```python
from build123d import *

# Parameters (mm, degrees)
SKETCH1_W           = 30.65
SKETCH1_H           = 12.1
BOSS_EXTRUDE1_DEPTH = 12.4
SKETCH2_R           = 2
SKETCH2_W           = 1.2
SKETCH2_H           = 4.3
CUT_EXTRUDE1_DEPTH  = 10
SKETCH3_R           = 0.425
CUT_EXTRUDE2_DEPTH  = 12.4
SKETCH4_W           = 30.65
SKETCH4_H           = 1.9
SKETCH4_W_2         = 17.6
SKETCH4_H_2         = 0.8
SKETCH4_W_3         = 6.5
SKETCH4_H_3         = 5.95
CUT_EXTRUDE3_DEPTH  = 10.1
CUT_EXTRUDE4_REACH  = 21.537
SKETCH6_W           = 6.5
SKETCH6_H           = 8.2
SKETCH7_W           = 15.65
SKETCH7_H           = 6.6
CUT_EXTRUDE5_DEPTH  = 6.35
CUT_EXTRUDE6_REACH  = 21.019
FILLET1_R           = 1.5
SKETCH10_W          = 3.4
SKETCH10_H          = 3
CUT_EXTRUDE7_DEPTH  = 4.8
SKETCH11_W          = 3.4
SKETCH11_H          = 3
CUT_EXTRUDE8_DEPTH  = 9.5
FILLET2_R           = 1.5
SKETCH12_R          = 2.5
CUT_EXTRUDE9_DEPTH  = 0.5
CUT_EXTRUDE10_REACH = 22.15
SKETCH13_W          = 0.8
SKETCH13_H          = 1.6
SKETCH13_H_2        = 4.5
FILLET3_R           = 0.25
SKETCH14_R          = 0.725
CUT_EXTRUDE11_DEPTH = 1


with BuildPart() as part:
    # Sketch1 → Boss-Extrude1 (new body)
    with BuildSketch(Plane(origin=(0, 0, 0), x_dir=(1, 0, 0), z_dir=(0, 1, 0))):
        Rectangle(SKETCH1_W, SKETCH1_H)
    extrude(amount=BOSS_EXTRUDE1_DEPTH)

    # Sketch2 → Cut-Extrude1 (cut)
    with BuildSketch(Plane.XY.offset(6.05)):
        with Locations((-12.5, 6.4)):
            Circle(SKETCH2_R)
        with Locations(Location((12.5, 6.4, 0), (0, 0, 180))):
            Circle(SKETCH2_R)
        with Locations((-7.3, 6.2)):
            Rectangle(SKETCH2_W, SKETCH2_H)
        with Locations((7.3, 6.2)):
            Rectangle(SKETCH2_W, SKETCH2_H)
    extrude(amount=-CUT_EXTRUDE1_DEPTH, mode=Mode.SUBTRACT)

    # Sketch3 → Cut-Extrude2 (cut)
    with BuildSketch(Plane.XY.offset(6.05)):
        with Locations((-5.1, 7.675)):
            Circle(SKETCH3_R)
        with Locations((-2.55, 7.675)):
            Circle(SKETCH3_R)
        with Locations((0, 7.675)):
            Circle(SKETCH3_R)
        with Locations((2.55, 7.675)):
            Circle(SKETCH3_R)
        with Locations((5.1, 7.675)):
            Circle(SKETCH3_R)
        with Locations((-3.825, 4.725)):
            Circle(SKETCH3_R)
        with Locations((-1.275, 4.725)):
            Circle(SKETCH3_R)
        with Locations((1.275, 4.725)):
            Circle(SKETCH3_R)
        with Locations((3.825, 4.725)):
            Circle(SKETCH3_R)
    extrude(amount=-CUT_EXTRUDE2_DEPTH, mode=Mode.SUBTRACT)

    # Sketch4 → Cut-Extrude3 (cut)
    with BuildSketch(Plane(origin=(0, 0, -6.05), x_dir=(-1, 0, 0), z_dir=(0, 0, -1))):
        with Locations((0, 11.45)):
            Rectangle(SKETCH4_W, SKETCH4_H)
        with Locations((0, 0.4)):
            Rectangle(SKETCH4_W_2, SKETCH4_H_2)
        with Locations((12.075, 5.875)):
            Rectangle(SKETCH4_W_3, SKETCH4_H_3)
        with Locations((-12.075, 5.875)):
            Rectangle(SKETCH4_W_3, SKETCH4_H_3)
    extrude(amount=-CUT_EXTRUDE3_DEPTH, mode=Mode.SUBTRACT)

    # Sketch6 → Cut-Extrude4 (cut, up to next)
    with BuildSketch(Plane(origin=(0, 10.5, 0), x_dir=(1, 0, 0), z_dir=(0, 1, 0)), mode=Mode.PRIVATE) as cut_extrude4_sk1:
        with Locations((12.075, 1.95)):
            Rectangle(SKETCH6_W, SKETCH6_H)
    cut_extrude4_tool1 = extrude(cut_extrude4_sk1.sketch, amount=-CUT_EXTRUDE4_REACH, mode=Mode.PRIVATE) & part.part
    # Sketch6 → Cut-Extrude4 (cut, up to next)
    with BuildSketch(Plane(origin=(0, 10.5, 0), x_dir=(1, 0, 0), z_dir=(0, 1, 0)), mode=Mode.PRIVATE) as cut_extrude4_sk2:
        with Locations((-12.075, 1.95)):
            Rectangle(SKETCH6_W, SKETCH6_H)
    cut_extrude4_tool2 = extrude(cut_extrude4_sk2.sketch, amount=-CUT_EXTRUDE4_REACH, mode=Mode.PRIVATE) & part.part
    add(cut_extrude4_tool1.solids().sort_by_distance((12.075, 10.5, -1.95))[0], mode=Mode.SUBTRACT)
    add(cut_extrude4_tool2.solids().sort_by_distance((-12.075, 10.5, -1.95))[0], mode=Mode.SUBTRACT)

    # Sketch7 → Cut-Extrude5 (cut)
    with BuildSketch(Plane(origin=(0, 0, -6.05), x_dir=(-1, 0, 0), z_dir=(0, 0, -1))):
        with Locations((0, 6.2)):
            Rectangle(SKETCH7_W, SKETCH7_H)
    extrude(amount=-CUT_EXTRUDE5_DEPTH, mode=Mode.SUBTRACT)

    # Sketch8 → Cut-Extrude6 (cut, up to next)
    with BuildSketch(Plane(origin=(0, 2.9, 0), x_dir=(1, 0, 0), z_dir=(0, 1, 0)), mode=Mode.PRIVATE) as cut_extrude6_sk1:
        with BuildLine():
            Line((-10.795, 3.45), (-10.795, 1.25))
            ThreePointArc((-10.795, 1.25), (-12.495, -0.45), (-14.195, 1.25))
            Line((-14.195, 1.25), (-14.195, 3.45))
            ThreePointArc((-14.195, 3.45), (-12.495, 5.15), (-10.795, 3.45))
        make_face()
    cut_extrude6_tool1 = extrude(cut_extrude6_sk1.sketch, amount=-CUT_EXTRUDE6_REACH, mode=Mode.PRIVATE) & part.part
    # Sketch8 → Cut-Extrude6 (cut, up to next)
    with BuildSketch(Plane(origin=(0, 2.9, 0), x_dir=(1, 0, 0), z_dir=(0, 1, 0)), mode=Mode.PRIVATE) as cut_extrude6_sk2:
        with BuildLine():
            Line((10.795, 3.45), (10.795, 1.25))
            ThreePointArc((10.795, 1.25), (12.495, -0.45), (14.195, 1.25))
            Line((14.195, 1.25), (14.195, 3.45))
            ThreePointArc((14.195, 3.45), (12.495, 5.15), (10.795, 3.45))
        make_face()
    cut_extrude6_tool2 = extrude(cut_extrude6_sk2.sketch, amount=-CUT_EXTRUDE6_REACH, mode=Mode.PRIVATE) & part.part
    add(cut_extrude6_tool1.solids().sort_by_distance((-12.495, 2.9, -2.35))[0], mode=Mode.SUBTRACT)
    add(cut_extrude6_tool2.solids().sort_by_distance((12.495, 2.9, -2.35))[0], mode=Mode.SUBTRACT)

    # Fillet1
    fillet1_edges = [part.edges().sort_by_distance(p)[0] for p in [
        (8.825, 10.5, -1.95),
        (-8.825, 10.5, -1.95),
    ]]
    fillet(fillet1_edges, radius=FILLET1_R)

    # Sketch10 → Cut-Extrude7 (cut)
    with BuildSketch(Plane(origin=(0, 0, -6.05), x_dir=(-1, 0, 0), z_dir=(0, 0, -1))):
        with Locations((-12.5, 2.9)):
            Rectangle(SKETCH10_W, SKETCH10_H)
    cut_extrude7 = extrude(amount=-CUT_EXTRUDE7_DEPTH, mode=Mode.SUBTRACT)

    # Sketch11 → Cut-Extrude8 (cut)
    with BuildSketch(Plane.XY.offset(6.05)):
        with Locations((12.5, 0)):
            Rectangle(SKETCH11_W, SKETCH11_H)
    cut_extrude8 = extrude(amount=-CUT_EXTRUDE8_DEPTH, mode=Mode.SUBTRACT)

    # Mirror3: Cut-Extrude7, Cut-Extrude8 across plane
    add(cut_extrude7.mirror(Plane(origin=(0, 0, 0), x_dir=(0, 0, 1), z_dir=(1, 0, 0))), mode=Mode.SUBTRACT)
    add(cut_extrude8.mirror(Plane(origin=(0, 0, 0), x_dir=(0, 0, 1), z_dir=(1, 0, 0))), mode=Mode.SUBTRACT)

    # Fillet2
    fillet2_edges = [part.edges().sort_by_distance(p)[0] for p in [
        (15.325, 12.4, 5.05),
        (-15.325, 12.4, 5.05),
    ]]
    fillet(fillet2_edges, radius=FILLET2_R)

    # Sketch12 → Cut-Extrude9 (cut)
    with BuildSketch(Plane.XY.offset(6.05)):
        with Locations((-12.5, 6.4)):
            Circle(SKETCH12_R)
        with Locations((12.5, 6.4)):
            Circle(SKETCH12_R)
    extrude(amount=-CUT_EXTRUDE9_DEPTH, mode=Mode.SUBTRACT)

    # Sketch13 → Cut-Extrude10 (cut, up to next)
    with BuildSketch(Plane.XZ.offset(-0.8), mode=Mode.PRIVATE) as cut_extrude10_sk1:
        with Locations((5.095, -5.25)):
            Rectangle(SKETCH13_W, SKETCH13_H)
    cut_extrude10_tool1 = extrude(cut_extrude10_sk1.sketch, amount=-CUT_EXTRUDE10_REACH, mode=Mode.PRIVATE) & part.part
    # Sketch13 → Cut-Extrude10 (cut, up to next)
    with BuildSketch(Plane.XZ.offset(-0.8), mode=Mode.PRIVATE) as cut_extrude10_sk2:
        with Locations((1.275, -3.8)):
            Rectangle(SKETCH13_W, SKETCH13_H_2)
    cut_extrude10_tool2 = extrude(cut_extrude10_sk2.sketch, amount=-CUT_EXTRUDE10_REACH, mode=Mode.PRIVATE) & part.part
    # Sketch13 → Cut-Extrude10 (cut, up to next)
    with BuildSketch(Plane.XZ.offset(-0.8), mode=Mode.PRIVATE) as cut_extrude10_sk3:
        with Locations((3.825, -3.8)):
            Rectangle(SKETCH13_W, SKETCH13_H_2)
    cut_extrude10_tool3 = extrude(cut_extrude10_sk3.sketch, amount=-CUT_EXTRUDE10_REACH, mode=Mode.PRIVATE) & part.part
    # Sketch13 → Cut-Extrude10 (cut, up to next)
    with BuildSketch(Plane.XZ.offset(-0.8), mode=Mode.PRIVATE) as cut_extrude10_sk4:
        with Locations((2.545, -5.25)):
            Rectangle(SKETCH13_W, SKETCH13_H)
    cut_extrude10_tool4 = extrude(cut_extrude10_sk4.sketch, amount=-CUT_EXTRUDE10_REACH, mode=Mode.PRIVATE) & part.part
    # Sketch13 → Cut-Extrude10 (cut, up to next)
    with BuildSketch(Plane.XZ.offset(-0.8), mode=Mode.PRIVATE) as cut_extrude10_sk5:
        with Locations((-1.275, -3.8)):
            Rectangle(SKETCH13_W, SKETCH13_H_2)
    cut_extrude10_tool5 = extrude(cut_extrude10_sk5.sketch, amount=-CUT_EXTRUDE10_REACH, mode=Mode.PRIVATE) & part.part
    # Sketch13 → Cut-Extrude10 (cut, up to next)
    with BuildSketch(Plane.XZ.offset(-0.8), mode=Mode.PRIVATE) as cut_extrude10_sk6:
        with Locations((-0.005, -5.25)):
            Rectangle(SKETCH13_W, SKETCH13_H)
    cut_extrude10_tool6 = extrude(cut_extrude10_sk6.sketch, amount=-CUT_EXTRUDE10_REACH, mode=Mode.PRIVATE) & part.part
    # Sketch13 → Cut-Extrude10 (cut, up to next)
    with BuildSketch(Plane.XZ.offset(-0.8), mode=Mode.PRIVATE) as cut_extrude10_sk7:
        with Locations((-3.825, -3.8)):
            Rectangle(SKETCH13_W, SKETCH13_H_2)
    cut_extrude10_tool7 = extrude(cut_extrude10_sk7.sketch, amount=-CUT_EXTRUDE10_REACH, mode=Mode.PRIVATE) & part.part
    # Sketch13 → Cut-Extrude10 (cut, up to next)
    with BuildSketch(Plane.XZ.offset(-0.8), mode=Mode.PRIVATE) as cut_extrude10_sk8:
        with Locations((-2.555, -5.25)):
            Rectangle(SKETCH13_W, SKETCH13_H)
    cut_extrude10_tool8 = extrude(cut_extrude10_sk8.sketch, amount=-CUT_EXTRUDE10_REACH, mode=Mode.PRIVATE) & part.part
    # Sketch13 → Cut-Extrude10 (cut, up to next)
    with BuildSketch(Plane.XZ.offset(-0.8), mode=Mode.PRIVATE) as cut_extrude10_sk9:
        with Locations((-5.095, -5.25)):
            Rectangle(SKETCH13_W, SKETCH13_H)
    cut_extrude10_tool9 = extrude(cut_extrude10_sk9.sketch, amount=-CUT_EXTRUDE10_REACH, mode=Mode.PRIVATE) & part.part
    add(cut_extrude10_tool1.solids().sort_by_distance((5.095, 0.8, -5.25))[0], mode=Mode.SUBTRACT)
    add(cut_extrude10_tool2.solids().sort_by_distance((1.275, 0.8, -3.8))[0], mode=Mode.SUBTRACT)
    add(cut_extrude10_tool3.solids().sort_by_distance((3.825, 0.8, -3.8))[0], mode=Mode.SUBTRACT)
    add(cut_extrude10_tool4.solids().sort_by_distance((2.545, 0.8, -5.25))[0], mode=Mode.SUBTRACT)
    add(cut_extrude10_tool5.solids().sort_by_distance((-1.275, 0.8, -3.8))[0], mode=Mode.SUBTRACT)
    add(cut_extrude10_tool6.solids().sort_by_distance((-0.005, 0.8, -5.25))[0], mode=Mode.SUBTRACT)
    add(cut_extrude10_tool7.solids().sort_by_distance((-3.825, 0.8, -3.8))[0], mode=Mode.SUBTRACT)
    add(cut_extrude10_tool8.solids().sort_by_distance((-2.555, 0.8, -5.25))[0], mode=Mode.SUBTRACT)
    add(cut_extrude10_tool9.solids().sort_by_distance((-5.095, 0.8, -5.25))[0], mode=Mode.SUBTRACT)

    # Fillet3
    # the kernel refuses this fillet: 0.25 mm, written as the material it takes off along each edge
    with BuildSketch(Plane(origin=(5.495, 0.175, -6.05), x_dir=(1, 0, 0), z_dir=(0, 1, 0))) as fillet3_piece_1:
        with BuildLine():
            CenterArc((FILLET3_R, -FILLET3_R), FILLET3_R, 90, 90)
            Line((0, -FILLET3_R), (0, 0))
            Line((0, 0), (FILLET3_R, 0))
        make_face()
    extrude(amount=3.35, mode=Mode.SUBTRACT)
    with BuildSketch(Plane(origin=(4.695, 0.175, -6.05), x_dir=(-1, 0, 0), z_dir=(0, 1, 0)), Plane(origin=(-4.225, 0.175, -6.05), x_dir=(-1, 0, 0), z_dir=(0, 1, 0)), Plane(origin=(-3.425, 0.175, -6.05), x_dir=(0, 0, 1), z_dir=(0, 1, 0)), Plane(origin=(-2.955, 0.175, -6.05), x_dir=(-1, 0, 0), z_dir=(0, 1, 0)), Plane(origin=(-2.155, 0.175, -6.05), x_dir=(0, 0, 1), z_dir=(0, 1, 0)), Plane(origin=(-1.675, 0.175, -6.05), x_dir=(-1, 0, 0), z_dir=(0, 1, 0)), Plane(origin=(-0.875, 0.175, -6.05), x_dir=(0, 0, 1), z_dir=(0, 1, 0)), Plane(origin=(-0.405, 0.175, -6.05), x_dir=(-1, 0, 0), z_dir=(0, 1, 0)), Plane(origin=(0.395, 0.175, -6.05), x_dir=(0, 0, 1), z_dir=(0, 1, 0)), Plane(origin=(0.875, 0.175, -6.05), x_dir=(-1, 0, 0), z_dir=(0, 1, 0)), Plane(origin=(1.675, 0.175, -6.05), x_dir=(0, 0, 1), z_dir=(0, 1, 0)), Plane(origin=(-5.495, 0.175, -6.05), x_dir=(-1, 0, 0), z_dir=(0, 1, 0)), Plane(origin=(-4.695, 0.175, -6.05), x_dir=(0, 0, 1), z_dir=(0, 1, 0)), Plane(origin=(3.425, 0.175, -6.05), x_dir=(-1, 0, 0), z_dir=(0, 1, 0)), Plane(origin=(4.225, 0.175, -6.05), x_dir=(0, 0, 1), z_dir=(0, 1, 0)), Plane(origin=(2.145, 0.175, -6.05), x_dir=(-1, 0, 0), z_dir=(0, 1, 0)), Plane(origin=(2.945, 0.175, -6.05), x_dir=(0, 0, 1), z_dir=(0, 1, 0))) as fillet3_piece_2:
        with BuildLine():
            CenterArc((FILLET3_R, FILLET3_R), FILLET3_R, 180, 90)
            Line((0, FILLET3_R), (0, 0))
            Line((0, 0), (FILLET3_R, 0))
        make_face()
    extrude(amount=3.35, mode=Mode.SUBTRACT)

    # Sketch14 → Cut-Extrude11 (cut)
    with BuildSketch(Plane(origin=(0, 0, 0.3), x_dir=(-1, 0, 0), z_dir=(0, 0, -1))):
        with Locations((-2.55, 7.675)):
            Circle(SKETCH14_R)
        with Locations((-5.1, 7.675)):
            Circle(SKETCH14_R)
        with Locations((0, 7.675)):
            Circle(SKETCH14_R)
        with Locations((2.55, 7.675)):
            Circle(SKETCH14_R)
        with Locations((5.1, 7.675)):
            Circle(SKETCH14_R)
        with Locations((3.825, 4.725)):
            Circle(SKETCH14_R)
        with Locations((1.275, 4.725)):
            Circle(SKETCH14_R)
        with Locations((-1.275, 4.725)):
            Circle(SKETCH14_R)
        with Locations((-3.825, 4.725)):
            Circle(SKETCH14_R)
    extrude(amount=-CUT_EXTRUDE11_DEPTH, mode=Mode.SUBTRACT)


solid = part.part
```
Input: part model. Units: mm. Frame: model coordinates. A direction names the side the tool comes from. Round coordinates to 2 decimals unless told otherwise and drop trailing zeros. Loops run counter-clockwise (first coordinate to the right, second up) from the corner with the lowest first, then second, coordinate; pieces in that order, holes last. Notation, with made-up numbers: (18, 48.5) -> (24, 48.5) arc R18 ccw to (24, 66.5) -> close; hole circle Ø8 at (86.5, -5.5). An arc over 180 degrees is marked (long way). Use one line per item in the form item = value. Start each with the question number.
Item 1: Section query D-D on y = 10. Return the cut outline in (x, z) (3 decimals), then the cut area to 3 significant figures.
Item 2: Section query B-B on x = 12.5. Return the cut outline in (y, z), then the cut area to 3 significant figures.
Item 3: Set-up query: faces 1 (the face through (10.5, 4.9, 5.8)), 2 (the face through (4.225, 2, -4)), 3 (the face through (-12.5, 1.4, -5.3)). Return all of +Z, -Z, +X, -X, +Y, -Y with unobstructed straight access to the full face (end or side cutting, diameter ignored); none if empty.
Item 4: Material intervals for L1, parallel to X at y = 8.25, z = 3.75 (3 decimals); L2, parallel to X at y = 4, z = -1.5 (3 decimals); L3, parallel to X at y = 6, z = -3 (3 decimals), sorted ascending. Write a range as from..to.
Item 5: Section query C-C on y = 6.4. Count the separate pieces of the cut face and the enclosed holes in it, then the cut area to 3 significant figures.
Item 6: Contact query for flat-ended pins moving along their axis: pin 1 Ø0.8 at (x, y) = (10.5, 9.5) entering from -Z; pin 2 Ø6 at (y, z) = (8.5, 3.5) entering from -X (3 decimals); pin 3 Ø3 at (x, y) = (12.5, 6.4) entering from -Z; pin 4 Ø5 at (y, z) = (10, -4) entering from -X (3 decimals). Output: stop coordinate, or through.
Item 7: Mould query, pull axis X, two halves, no side actions, for faces 4 (the face through (0, 0, 5)), 5 (the face through (7.9, 6, 1)). Classes: pulls with the +X half, pulls with the -X half, needs draft (parallel to the pull), parting line crosses it, or undercut.
Item 8: Section query A-A on x = -7. Return the cut outline in (y, z), then the cut area to 3 significant figures.
Ans:
q1.outline = (-15.325, 2.15) -> (-8.443, 2.15) -> (-8.443, -6.05) -> (8.443, -6.05) -> (8.443, 2.15) -> (15.325, 2.15) -> (15.325, 6.05) -> (-15.325, 6.05) -> close
q1.area = 258 mm^2
q2.outline = (0, -6.05) -> (1.4, -6.05) -> (1.4, -5.15) -> (0, -5.15) -> close; (1.5, 0.45) -> (2.9, 0.45) -> (2.9, 4.05) -> (4.4, 4.05) -> (4.4, 5.55) -> (3.9, 5.55) -> (3.9, 6.05) -> (1.5, 6.05) -> close; (8.4, 4.05) -> (8.85, 4.05) -> (8.85, 2.15) -> (10.5, 2.15) -> (10.5, 4.05) -> (12.4, 4.05) -> (12.4, 6.05) -> (8.9, 6.05) -> (8.9, 5.55) -> (8.4, 5.55) -> close
q2.area = 22.7 mm^2
q3.face_1 = +Z
q3.face_2 = -Z, -Y
q3.face_3 = +Z, -Z, +Y
q4.L1 = -8.825..-7.9, -6.7..6.7, 7.9..8.825
q4.L2 = -8.825..-7.825, 7.825..8.825
q4.L3 = -8.825..-7.9, 7.9..8.825
q5.separate_pieces = 5
q5.enclosed_holes = 0
q5.area = 109 mm^2
q6.pin_1 = 2.15
q6.pin_2 = -15.325
q6.pin_3 = through
q6.pin_4 = -8.825
q7.face_4 = needs draft
q7.face_5 = undercut
q8.outline = (0, 4.05) -> (0.8, 4.05) -> (0.8, -6.05) -> (2.9, -6.05) -> (2.9, 0.3) -> (4.05, 0.3) -> (4.05, 6.05) -> (0, 6.05) -> close; (8.35, 0.3) -> (9.5, 0.3) -> (9.5, -6.05) -> (10.5, -6.05) -> (10.5, 4.05) -> (12.4, 4.05) -> (12.4, 6.05) -> (8.35, 6.05) -> close
q8.area = 56.1 mm^2
